from build123d import *

# Parameters (mm, degrees)
SKETCH1_R                 = 35
BOSS_EXTRUDE1_DEPTH       = 25
SKETCH2_R                 = 15
BOSS_EXTRUDE2_DEPTH       = 90
FILLET1_R                 = 10
SKETCH3_W                 = 35
SKETCH3_H                 = 50
SKETCH3_R                 = 2
BOSS_EXTRUDE3_DEPTH       = 5
REVOLVE1_ANGLE            = 180
BOSS_EXTRUDE4_OUTLINE_R   = 33.541019662
BOSS_EXTRUDE4_OUTLINE_R_2 = 30
BOSS_EXTRUDE4_DEPTH       = 20


# Read off the part's stored shape, not the designer's step: Boss-Extrude4
with BuildPart() as part:
    # Sketch1 → Boss-Extrude1 (new body)
    with BuildSketch(Plane.XY):
        Circle(SKETCH1_R)
    extrude(amount=BOSS_EXTRUDE1_DEPTH)

    # Sketch2 → Boss-Extrude2 (add)
    with BuildSketch(Plane(origin=(0, 0, 0), x_dir=(-1, 0, 0), z_dir=(0, 0, -1))):
        with Locations(Location((0, 0, 0), (0, 0, 180))):
            Circle(SKETCH2_R)
    extrude(amount=BOSS_EXTRUDE2_DEPTH)

    # Fillet1
    fillet1_edges = [part.edges().sort_by_distance(p)[0] for p in [
        (-35, 0, 0),
        (-15, 0, 0),
    ]]
    fillet(fillet1_edges, radius=FILLET1_R - 0.0001)  # a hair under: the kernel refuses the full size

    # Sketch3 → Boss-Extrude3 (add, symmetric)
    with BuildSketch(Plane(origin=(0, 0, 0), x_dir=(1, 0, 0), z_dir=(0, 1, 0))):
        with Locations((0, -50)):
            Rectangle(SKETCH3_W, SKETCH3_H)
        with Locations(Location((-10, -35.1, 0), (0, 0, 270))):
            Circle(SKETCH3_R, mode=Mode.SUBTRACT)
        with Locations(Location((10, -35.1, 0), (0, 0, 270))):
            Circle(SKETCH3_R, mode=Mode.SUBTRACT)
        with Locations(Location((10, -65.1, 0), (0, 0, 270))):
            Circle(SKETCH3_R, mode=Mode.SUBTRACT)
        with Locations(Location((-10, -65.1, 0), (0, 0, 270))):
            Circle(SKETCH3_R, mode=Mode.SUBTRACT)
    extrude(amount=BOSS_EXTRUDE3_DEPTH, both=True)

    # Sketch4 → Revolve1 (revolve)
    with BuildSketch(Plane(origin=(0, 0, 0), x_dir=(1, 0, 0), z_dir=(0, 1, 0))):
        with BuildLine():
            Line((0, 150), (0, 153.541019662))
            ThreePointArc((0, 153.541019662), (-33.541019662, 120), (0, 86.458980338))
            Line((0, 86.458980338), (0, 90))
            ThreePointArc((0, 90), (-30, 120), (0, 150))
        make_face()
    revolve(axis=Axis((0, 0, -90), (0, 0, 1)), revolution_arc=REVOLVE1_ANGLE)

    # Boss-Extrude4 outline → Boss-Extrude4 (add)
    with BuildSketch(Plane(origin=(0, 0, 0), x_dir=(1, 0, 0), z_dir=(0, 1, 0))):
        with Locations((0, 120)):
            Circle(BOSS_EXTRUDE4_OUTLINE_R)
        with Locations((0, 120)):
            Circle(BOSS_EXTRUDE4_OUTLINE_R_2, mode=Mode.SUBTRACT)
    extrude(amount=BOSS_EXTRUDE4_DEPTH)


solid = part.part
Here's how the part is built. I have some questions about the finished solid (model axes, mm). A direction names the side the tool comes from. Give positions to 0.01 mm unless a question says otherwise; leave off trailing zeros. Order: outer loops, then holes, each group sorted by start corner. A loop starts at its lowest first (then second) coordinate and runs counter-clockwise, first axis right, second up. Notation, with made-up numbers: M 34.5,28 L 79.5,28 A26 cw 79.5,51 Z; hole C -13.5,72 d3. An arc over 180 degrees is marked long. Answer as a JSON object with one key per item and string values. Group by question number.
1) Suppose I cut it at A-A, the plane z = 35.1. Write out the boundary of the cut face in (x, y), plus the area to 3 significant figures.
2) We'd pull the mould along X, two halves only. Please class faces 5 (the flat face through (-25, 20, -103)), 6 (the cylindrical face through (11.352, -0.07, 63.626)), 7 (the cylindrical face through (-28, -21, 17)): pulls with the +X half, pulls with the -X half, needs draft (parallel to the pull), parting line crosses it, or undercut.
3) Please list where these lines run through material, in increasing order: L1, parallel to X at y = 0, z = 65; L2, parallel to Z at x = -21, y = -3; L3, parallel to Y at x = -3.5, z = 48. Write a range as [from, to].
4) Suppose I cut it at D-D, the plane x = 10. Count the separate pieces of the cut face and the enclosed holes in it, plus the area to 3 significant figures.
5) I'm going to push flat-ended pins straight in: pin 1 Ø1 at (y, z) = (-6, -100.5) entering from -X; pin 2 Ø17.5 at (x, z) = (-1, 43.5) entering from +Y; pin 3 Ø6 at (y, z) = (-19.5, -103.5) entering from +X. Where does each tip first touch, or does it pass through?
6) On a 3-axis mill with a long thin cutter (end or side, diameter ignored), from which of +Z, -Z, +X, -X, +Y, -Y can I reach the whole of each face in a straight line? I mean faces 1 (the flat face through (17.5, 0, 50)), 2 (the flat face through (0, 5, 50)), 3 (the cylindrical face through (8.06, -12.65, -49.44)), 4 (the flat face through (-17.5, 0, 50)). Say none if no direction works.
7) Suppose I cut it at C-C, the plane z = -120. Write out the boundary of the cut face in (x, y).
Results found:
{
 "1": {"outline": "M -17.5,-5 L -12,-5 L -12,5 L -17.5,5 Z; M -8,-5 L 8,-5 L 8,5 L -8,5 Z; M 12,-5 L 17.5,-5 L 17.5,5 L 12,5 Z", "area": "270 mm²"},
 "2": {"face 5": "needs draft", "face 6": "undercut", "face 7": "parting line crosses it"},
 "3": {"L1": "[-17.5, -12], [-8, 8], [12, 17.5]", "L2": "[-145.98, -141.21], [-98.79, -94.02], [-0.74, 25]", "L3": "[-5, 5]"},
 "4": {"separate pieces": "3", "enclosed holes": "0", "area": "4,580 mm²"},
 "5": {"pin 1": "x = -27", "pin 2": "y = 5", "pin 3": "x = 24.83"},
 "6": {"face 1": "+Z, +X, +Y, -Y", "face 2": "+Z, +X, -X, +Y", "face 3": "none", "face 4": "+Z, -X, +Y, -Y"},
 "7": {"outline": "M -33.54,0 A33.54 ccw 33.54,0 L 33.54,20 L 30,20 L 30,0 A30 cw -30,0 L -30,20 L -33.54,20 Z"}
}
